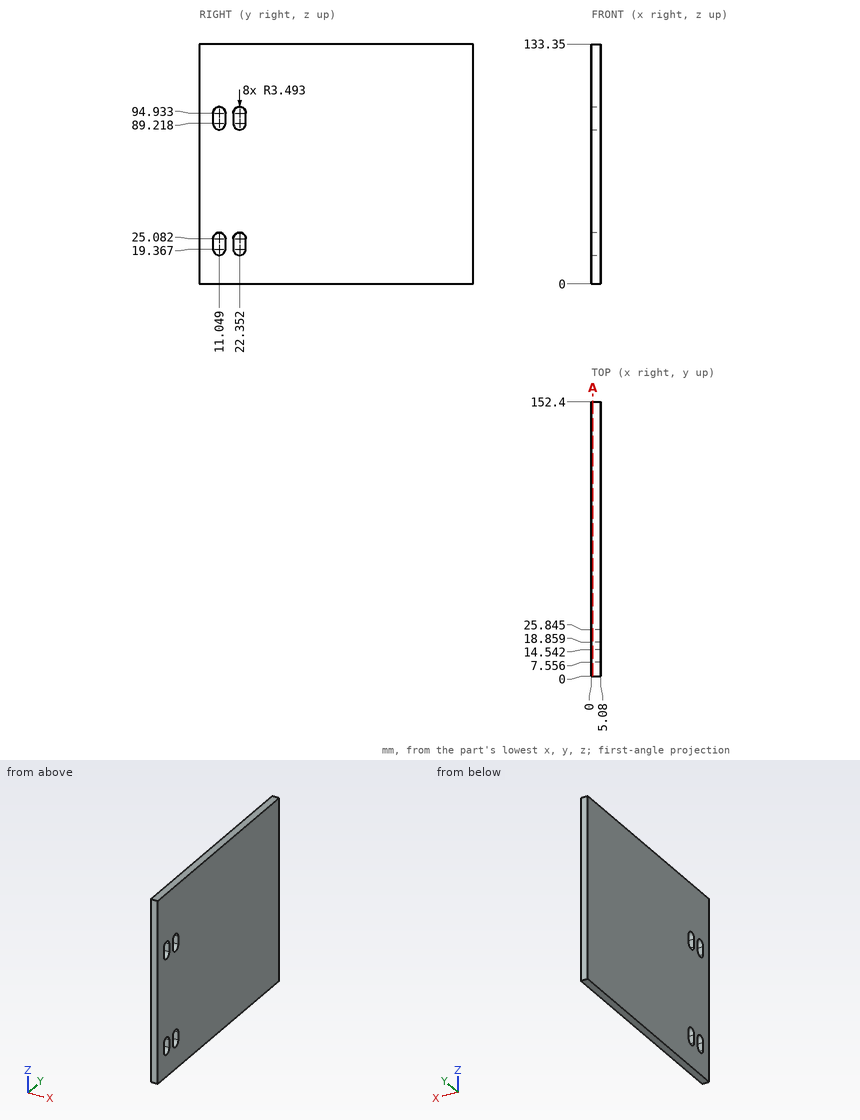
Input: dimensioned drawing with shaded views. Units: mm. Origin: part minimum x, y, z. Coordinates: 2 decimals unless noted, no trailing zeros. Answer in a Markdown table with one row per item.
Item 1: Ray query, L1, parallel to Y at x = 1.7, z = 21 (1 decimal); L2, parallel to Z at x = 3.7, y = 9.5; L3, parallel to Z at x = 1.5, y = 10.5. Return the intervals inside material, ascending.
Return value:
| item | result |
|---|---|
| L1 | y = 0 to 7.6, 14.5 to 18.9, 25.8 to 152.4 |
| L2 | z = 0 to 16.24, 28.21 to 86.09, 98.06 to 133.35 |
| L3 | z = 0 to 15.92, 28.53 to 85.77, 98.38 to 133.35 |
Item 2: Contact query for a flat-ended pin moving along its axis: P1, Ø3, axis at x = 1.5, z = 98, coming from the -Y side. Output: stop coordinate, or through.
Return value:
| item | result |
|---|---|
| P1 | stops at y = 0 |
Item 3: Section A-A on x = 0.8. State how many separate pieces and enclosed holes the cut face has, plus the area to 3 significant figures.
Return value:
| item | result |
|---|---|
| separate pieces | 1 |
| enclosed holes | 4 |
| area | 20,000 mm² |
